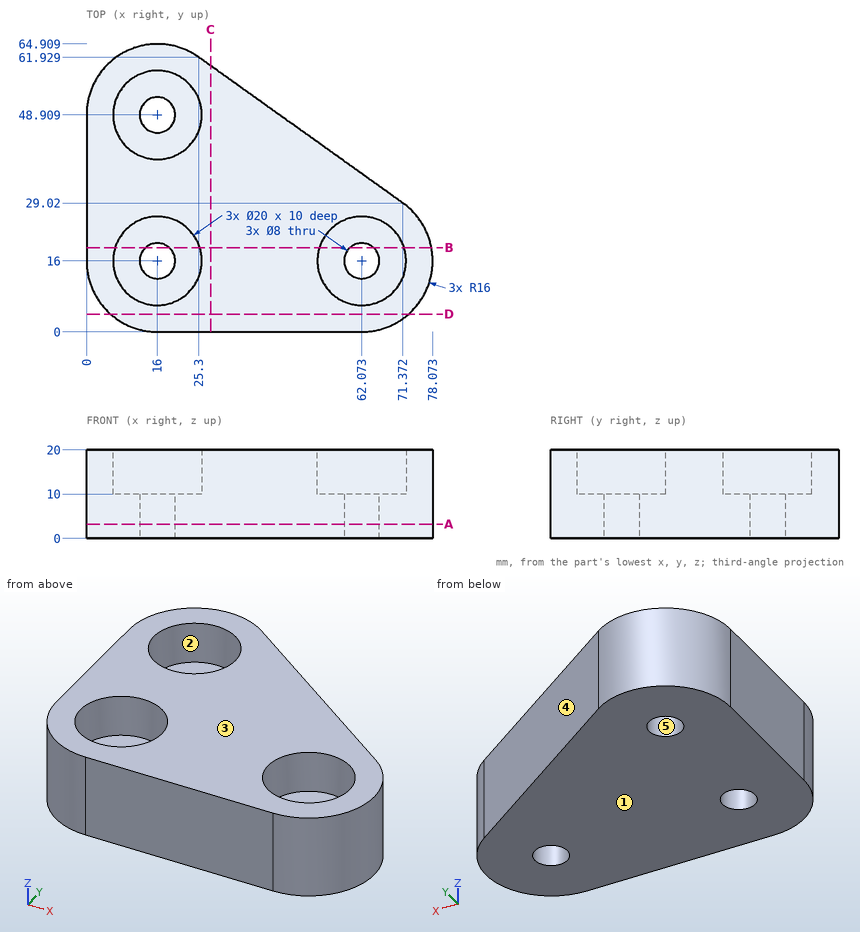
Can you work these out from the drawing? Everything is in mm from the part's minimum corner. A direction names the side the tool comes from. Give positions to 0.01 mm unless a question says otherwise; leave off trailing zeros. Loops run counter-clockwise (first coordinate to the right, second up) from the corner with the lowest first, then second, coordinate; pieces in that order, holes last. Notation, with made-up numbers: M 9,-18.75 L 27,-18.75 A26 cw 27,1.25 Z; hole C -8.5,61.5 d8. An arc over 180 degrees is marked long. Put each result on its own line as item: value. Start each with the question number.
(1) I want a section at C-C on x = 28. Please give me the cut outline in (y, z).
(2) For the marked faces 1 and 2, which set-ups out of +Z, -Z, +X, -X, +Y, -Y let a thin tool reach every point of the face, with its end or its side?
(3) I want a section at D-D on y = 4. Please give me the cut outline in (x, z) (1 decimal).
(4) I need wall thicknesses on line 1 along Y through (x, z) = (16, 6.75); line 2 along Y through (x, z) = (16, 13); line 3 along X through (y, z) = (15, 5.5) (1 decimal). Which ranges of each line are inside material? Lowest first, please. Write a range as [from, to].
(5) I want a section at A-A on z = 3.25. Please give me the cut outline in (x, y), then the cut area to 3 significant figures.
(6) I want a section at B-B on y = 19. Please give me the cut outline in (x, z) (1 decimal), then the cut area to 3 significant figures.
(7) Will these pins go through, and if not, where does the flat tip stop? pin 1 Ø10 at (y, z) = (8.5, 18) entering from +X; pin 2 Ø6 at (x, y) = (17, 47) entering from +Z; pin 3 Ø10 at (y, z) = (55.5, 15) entering from -X.
(8) If we mould it in two halves opening along X, with no side actions, what happens to the marked faces 3, 4 and 5? For each: +X half, -X half, draft (parallel to the pull), parting line (faces both ways), or undercut.
Answer block:
1. outline: M 0,0 L 60,0 L 60,20 L 0,20 Z
2. face 1: -Z, +X, -X, +Y, -Y
2. face 2: +Z
3. outline: M 5.4,0 L 72.7,0 L 72.7,20 L 5.4,20 Z
4. line 1: [0, 12], [20, 44.91], [52.91, 64.91]
4. line 2: [0, 6], [26, 38.91], [58.91, 64.91]
4. line 3: [0, 12.1], [19.9, 58.2], [65.9, 78]
5. outline: M 0,16 A16 ccw 16,0 L 62.07,0 A16 ccw 71.37,29.02 L 25.3,61.93 A16 ccw 0,48.91 Z; hole C 16,16 d8; hole C 16,48.91 d8; hole C 62.07,16 d8
5. area: 3,580 mm^2
6. outline: M 0,0 L 13.4,0 L 13.4,10 L 6.5,10 L 6.5,20 L 0,20 Z; M 18.6,0 L 59.4,0 L 59.4,10 L 52.5,10 L 52.5,20 L 25.5,20 L 25.5,10 L 18.6,10 Z; M 64.7,0 L 77.8,0 L 77.8,20 L 71.6,20 L 71.6,10 L 64.7,10 Z
6. area: 1,070 mm^2
7. pin 1: x = 77.88
7. pin 2: z = 10
7. pin 3: x = 0.08
8. face 3: draft
8. face 4: +X half
8. face 5: undercut
